Could you check a few things on this drawing? It's one solid part, dimensions in mm from its lowest x, y, z. A direction names the side the tool comes from. Round coordinates to 2 decimals unless told otherwise and drop trailing zeros. Write each loop counter-clockwise with the first axis right and the second up, starting at its lowest first coordinate (ties: lowest second). Pieces come first, ordered by that corner, then holes. Notation, with made-up numbers: (50.5, 5) - (97.5, 5) arc R21 ccw to (97.5, 42) - close; hole circle Ø4 at (17.25, -18). An arc over 180 degrees is marked (long way). Use one line per item in the form item = value. Start each with the question number.
1. I want a section at D-D, the plane y = 9.75. List the corners of the cut face in (x, z) for me.
2. Which directions (+Z, -Z, +X, -X, +Y, -Y) give clear straight access to the entire face, cutting with the end or side of a thin tool? Please do the marked faces 4 and 5.
3. If I drill on line 1 along Z through (x, y) = (12.7, 2.6); line 2 along Z through (x, y) = (12.7, 18.5); line 3 along X through (y, z) = (11.25, 10.75), over which ranges is the centre line in solid material (lowest first)?
4. I want a section at B-B, the plane x = 12.7. List the corners of the cut face in (y, z) for me, plus the area to 3 significant figures.
5. We'd pull the mould along Z, two halves only. Please class the marked faces 1, 2 and 3: +Z half, -Z half, draft (parallel to the pull), parting line (faces both ways), or undercut.
6. Will these pins go through, and if not, where does the flat tip stop? pin 1 (3 mm diameter, centred on y = 22, z = 18, fed in from +X); pin 2 (8 mm diameter, centred on x = 7.5, y = 16.5, fed in from +Z); pin 3 (5 mm diameter, centred on y = 22, z = 17.5, fed in from +X).
7. I want a section at C-C, the plane y = 1.75. List the corners of the cut face in (x, z) for me.
8. I want a section at A-A, the plane z = 12.7. List the corners of the cut face in (x, y) for me.
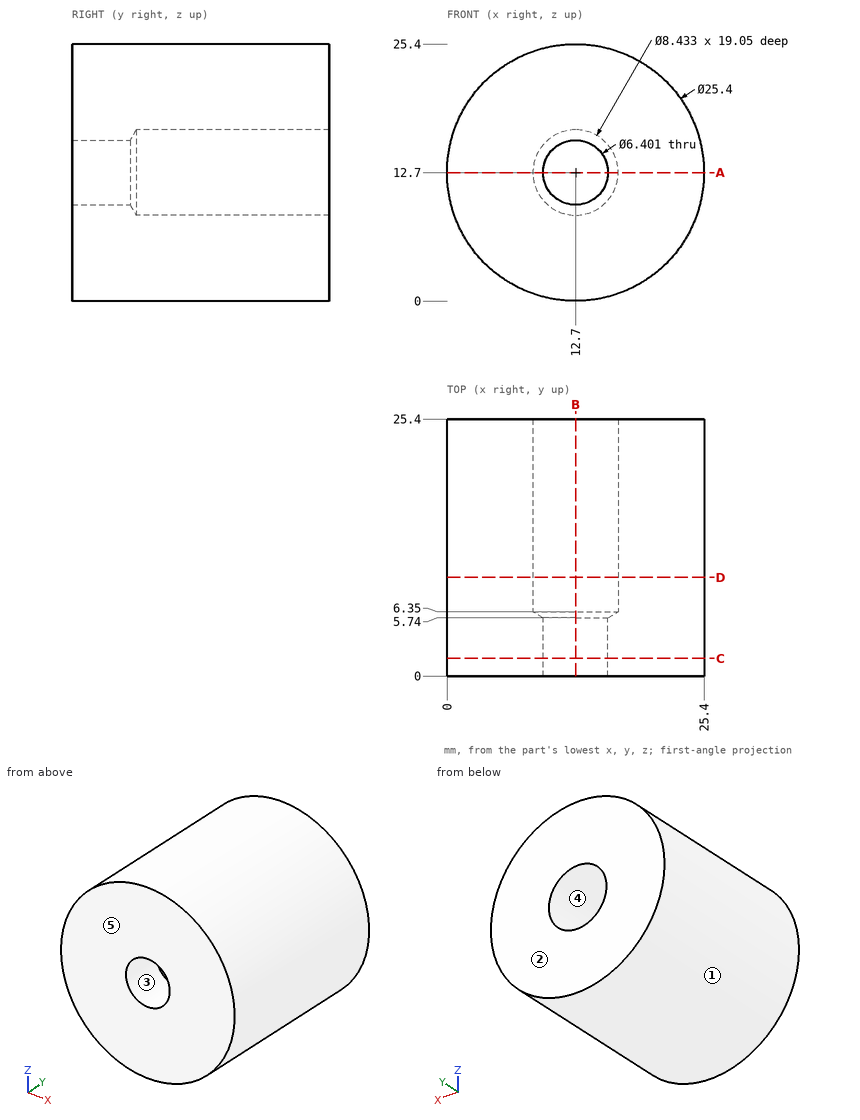
Model answer:
q1.outline = circle Ø25.4 at (12.7, 12.7); hole circle Ø8.43 at (12.7, 12.7)
q2.face_4 = +Y
q2.face_5 = +Z, -Z, +X, -X, -Y
q3.line_1 = 0 to 9.5, 15.9 to 25.4
q3.line_2 = 0 to 8.48, 16.92 to 25.4
q3.line_3 = 0.15 to 8.96, 16.44 to 25.25
q4.outline = (0, 0) - (25.4, 0) - (25.4, 8.48) - (6.35, 8.48) - (5.74, 9.5) - (0, 9.5) - close; (0, 15.9) - (5.74, 15.9) - (6.35, 16.92) - (25.4, 16.92) - (25.4, 25.4) - (0, 25.4) - close
q4.area = 443 mm2
q5.face_1 = parting line
q5.face_2 = draft
q5.face_3 = undercut
q6.pin_1 = 24.82
q6.pin_2 = 25.34
q6.pin_3 = 25.19
q7.outline = circle Ø25.4 at (12.7, 12.7); hole circle Ø6.4 at (12.7, 12.7)
q8.outline = (0, 0) - (9.5, 0) - (9.5, 5.74) - (8.48, 6.35) - (8.48, 25.4) - (0, 25.4) - close; (15.9, 0) - (25.4, 0) - (25.4, 25.4) - (16.92, 25.4) - (16.92, 6.35) - (15.9, 5.74) - close
